Drawing for the job (mm, zero at the part's lowest x, y, z). Round coordinates to 2 decimals unless told otherwise and drop trailing zeros. Loops run counter-clockwise (first coordinate to the right, second up) from the corner with the lowest first, then second, coordinate; pieces in that order, holes last. Notation, with made-up numbers: M 86,4.25 L 105,4.25 A19 cw 105,12.25 Z; hole C 0,22 d7. An arc over 180 degrees is marked long. Write each question's results on one line, items separated by ' | '.
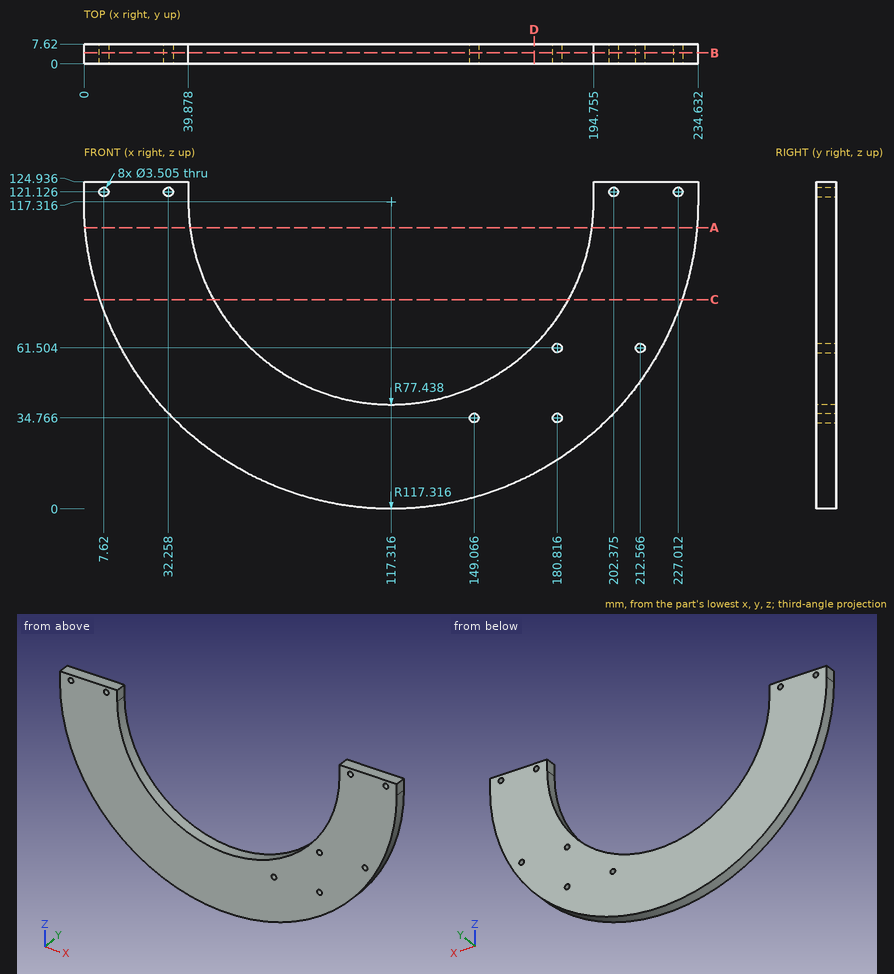
Item 1: Band-saw the part on D-D on x = 172. Give the cut face in (y, z) (1 decimal), and give its area (3 significant figures).
Filled sheet:
outline: M 0,13.5 L 7.6,13.5 L 7.6,62.5 L 0,62.5 Z | area: 373 mm^2
Item 2: Wall check: L1, parallel to X at y = 3.25, z = 71 (1 decimal); L2, parallel to X at y = 5, z = 92 (1 decimal); L3, parallel to Z at x = 82, y = 4.5. Give the ranges that are in metal, low to high.
Filled sheet:
L1: 9.5 to 55.3, 179.4 to 225.1 | L2: 2.8 to 44.1, 190.5 to 231.9 | L3: 5.44 to 48.4
Item 3: Band-saw the part on A-A on z = 107.5. Give the cut face in (x, y).
Filled sheet:
outline: M 0.41,0 L 40.5,0 L 40.5,7.62 L 0.41,7.62 Z; M 194.13,0 L 234.22,0 L 234.22,7.62 L 194.13,7.62 Z
Item 4: Band-saw the part on B-B on y = 4.25. Count the separate pieces of the cut face and the enclosed holes in it, and give its area (3 significant figures).
Filled sheet:
separate pieces: 1 | enclosed holes: 8 | area: 12,700 mm^2
Item 5: Drop flat-ended pins along their axis: P1, Ø1.5, axis at y = 1, z = 97, coming from the +X side; P2, Ø3, axis at x = 156, y = 6.5, coming from the -Z side; P3, Ø1.5, axis at x = 53.5, y = 2, coming from the -Z side. Give the stop position or say it passes through.
Filled sheet:
P1: x = 232.99 | P2: z = 6.05 | P3: z = 18.39
Item 6: Band-saw the part on C-C on z = 80. Give the cut face in (x, y), and give its area (3 significant figures).
Filled sheet:
outline: M 6.09,0 L 49.46,0 L 49.46,7.62 L 6.09,7.62 Z; M 185.17,0 L 228.54,0 L 228.54,7.62 L 185.17,7.62 Z | area: 661 mm^2
